The drawing under review shows one solid part. Ordinate dimensions are in mm from its lowest x, y, z. A direction names the side the tool comes from. Coordinates: 2 decimals unless noted, no trailing zeros. Write each loop counter-clockwise with the first axis right and the second up, starting at its lowest first coordinate (ties: lowest second). Pieces come first, ordered by that corner, then holes.
1) Add section B-B, the plane x = 21.5. State the section outline as (y, z) points.
2) For line 1 (Y direction, x = 13.5, z = 7); line 2 (Z direction, x = 7.5, y = 85); line 3 (X direction, y = 69, z = 9.5), list the stretches that pass through material, from the lowest coordinate up.
3) Mouldability with a two-part tool opening along X and no side actions: class the marked faces 3, 4, 5 and 6 as released by +X, released by -X, zero draft, split by the parting line, or undercut.
4) Add section D-D, the plane y = 81.5. State the section outline as (x, z) points.
5) Machinability: for the marked faces 1 and 2, which of the approach directions +Z, -Z, +X, -X, +Y, -Y give a long, thin tool a straight path to every point of the face, cutting with its end or side? Answer none if there is none.
6) Add section A-A, the plane y = 69. State the section outline as (x, z) points.
7) Add section C-C, the plane z = 7.5. State the section outline as (x, y) points, then the cut area to 3 significant figures.
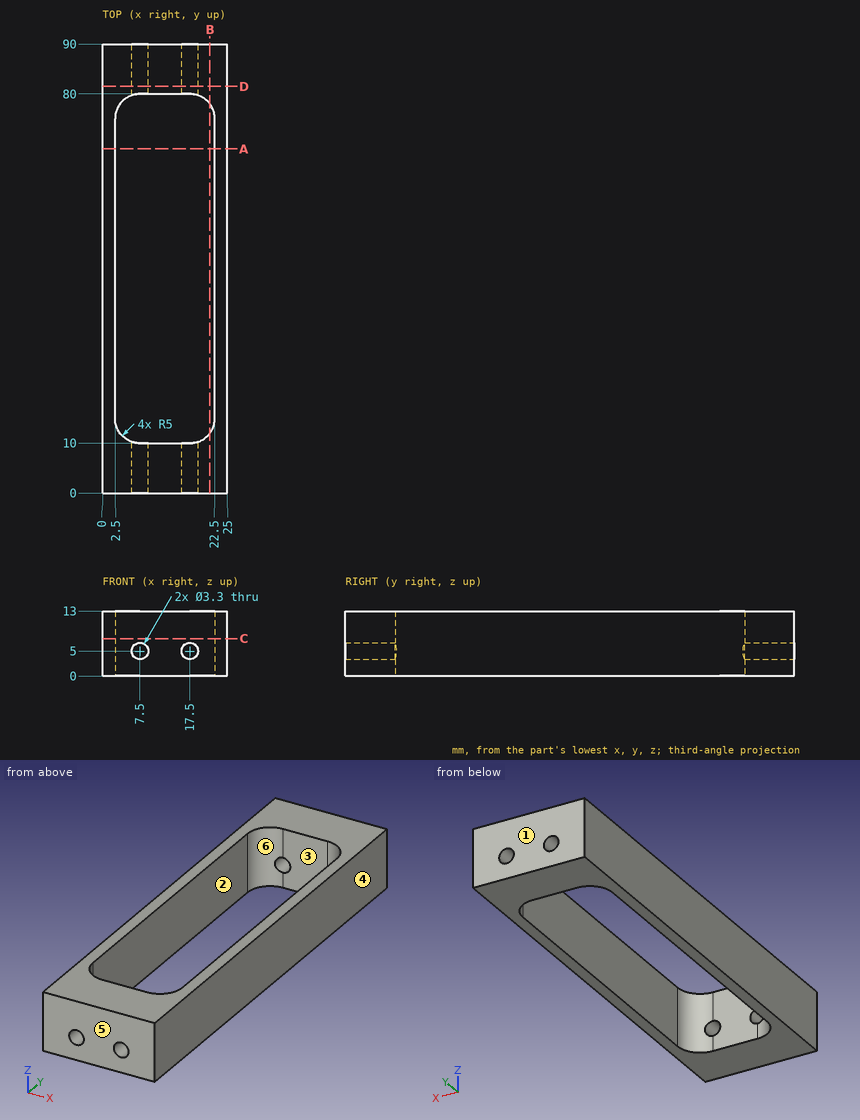
Geometry results:
1. outline: (0, 0) - (12, 0) - (12, 13) - (0, 13) - close; (78, 0) - (90, 0) - (90, 13) - (78, 13) - close
2. line 1: y = 0 to 10, 80 to 90
2. line 2: z = 0 to 3.35, 6.65 to 13
2. line 3: x = 0 to 2.5, 22.5 to 25
3. face 3: undercut
3. face 4: released by +X
3. face 5: zero draft
3. face 6: undercut
4. outline: (0, 0) - (25, 0) - (25, 13) - (0, 13) - close; hole circle Ø3.3 at (7.5, 5); hole circle Ø3.3 at (17.5, 5)
5. face 1: +Z, -Z, +X, -X, +Y
5. face 2: +Z, -Z
6. outline: (0, 0) - (2.5, 0) - (2.5, 13) - (0, 13) - close; (22.5, 0) - (25, 0) - (25, 13) - (22.5, 13) - close
7. outline: (0, 0) - (25, 0) - (25, 90) - (0, 90) - close; hole (2.5, 15) arc R5 ccw to (7.5, 10) - (17.5, 10) arc R5 ccw to (22.5, 15) - (22.5, 75) arc R5 ccw to (17.5, 80) - (7.5, 80) arc R5 ccw to (2.5, 75) - close
7. area: 871 mm2
